Input: dimensioned drawing with shaded views. Units: mm. Origin: part minimum x, y, z. Give positions to 0.01 mm unless a question says otherwise; leave off trailing zeros. Order: outer loops, then holes, each group sorted by start corner. A loop starts at its lowest first (then second) coordinate and runs counter-clockwise, first axis right, second up. Notation, with made-up numbers: (49, 47.5) - (66, 47.5) arc R25 cw to (66, 64.5) - close; hole circle Ø4 at (-18.5, -34). An arc over 180 degrees is marked (long way). Use a Markdown table: item, result.
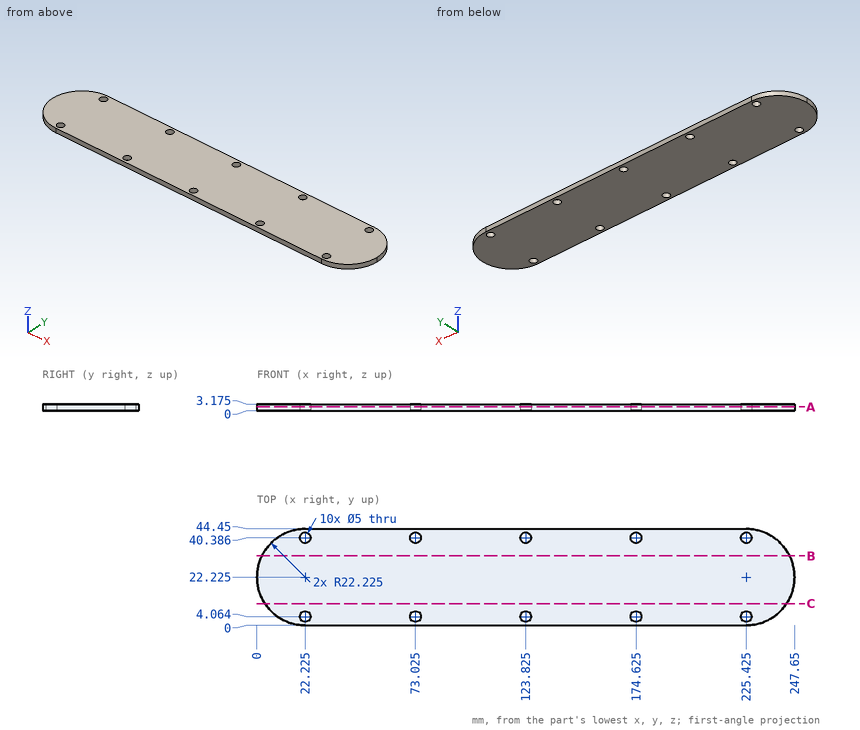
1. Pin query (flat end, axial travel): pin 1 (1.5 mm diameter, centred on y = 11, z = 1, fed in from +X); pin 2 (5.5 mm diameter, centred on x = 123.825, y = 40.386, fed in from +Z) (3 decimals); pin 3 (1 mm diameter, centred on y = 15.5, z = 0.5, fed in from +X); pin 4 (4 mm diameter, centred on x = 225.425, y = 4.064, fed in from +Z). Return the tip coordinate at first contact, or that it passes through.
Response:
| item | result |
|---|---|
| pin 1 | stops at x = 245.03 |
| pin 2 | stops at z = 3.175 |
| pin 3 | stops at x = 246.76 |
| pin 4 | passes through |
2. Section query B-B (y = 32). Return loops of the section in (x, z) (3 decimals).
Response:
| item | result |
|---|---|
| outline | (2.265, 0) - (245.385, 0) - (245.385, 3.175) - (2.265, 3.175) - close |
3. Section query A-A (z = 1.9). State how many separate pieces and enclosed holes the cut face has, then the cut area to 3 significant figures.
Response:
| item | result |
|---|---|
| separate pieces | 1 |
| enclosed holes | 10 |
| area | 10,400 mm^2 |
4. Material intervals for line 1 along Y through (x, z) = (123.5, 1.1); line 2 along X through (y, z) = (4, 0.9); line 3 along X through (y, z) = (36, 2.7), sorted ascending.
Response:
| item | result |
|---|---|
| line 1 | y = 0 to 1.59, 6.54 to 37.91, 42.86 to 44.45 |
| line 2 | x = 9.5 to 19.73, 24.72 to 70.53, 75.52 to 121.33, 126.32 to 172.13, 177.12 to 222.93, 227.92 to 238.15 |
| line 3 | x = 4.78 to 242.87 |
5. Section query C-C (y = 10). Return loops of the section in (x, z) (3 decimals).
Response:
| item | result |
|---|---|
| outline | (3.664, 0) - (243.986, 0) - (243.986, 3.175) - (3.664, 3.175) - close |
